Input: dimensioned drawing with shaded views. Units: mm. Origin: part minimum x, y, z. Round coordinates to 2 decimals unless told otherwise and drop trailing zeros. Loops run counter-clockwise (first coordinate to the right, second up) from the corner with the lowest first, then second, coordinate; pieces in that order, holes last. Notation, with made-up numbers: (81.25, -26.5) - (123.25, -26.5) arc R22 ccw to (123.25, 8.5) - close; hole circle Ø1 at (69.25, -26). An arc over 180 degrees is marked (long way). Answer as CSV lines item,"result".
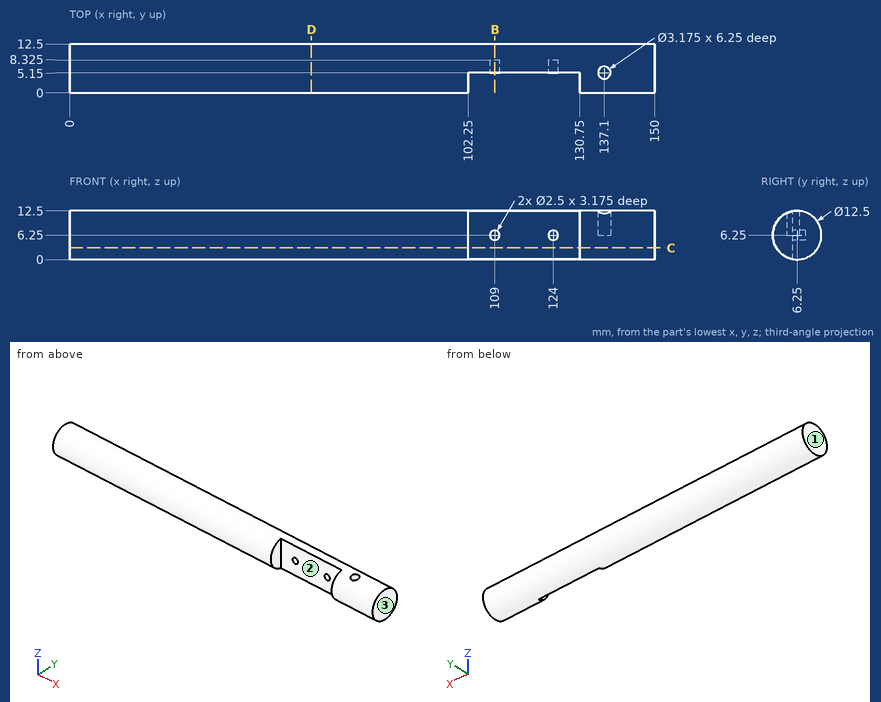
(1) Draft query along X for the marked faces 1, 2 and 3. Return one class per face: pulls with the +X half, pulls with the -X half, needs draft (parallel to the pull), parting line crosses it, or undercut.
Findings below:
face 1,"pulls with the -X half"
face 2,"undercut"
face 3,"pulls with the +X half"
(2) Material intervals for line 1 along Z through (x, y) = (109, 6.55); line 2 along X through (y, z) = (1.5, 6); line 3 along X through (y, z) = (5.25, 7.25), sorted ascending.
Findings below:
line 1,"0.01 to 5, 7.5 to 12.49"
line 2,"0 to 102.25, 130.75 to 150"
line 3,"0 to 108.25, 109.75 to 123.25, 124.75 to 135.52, 138.68 to 150"
(3) Section B-B (x = 109). Output: boundary loops of the cut face in (y, z) (3 decimals).
Findings below:
outline,"(5.15, 0.098) arc R6.25 ccw (long way) to (5.15, 12.402) - (5.15, 7.5) - (8.325, 7.5) - (8.325, 5) - (5.15, 5) - close"
(4) Section C-C (z = 3). Output: boundary loops of the cut face in (x, y), and give its area (3 significant figures).
Findings below:
outline,"(0, 0.91) - (102.25, 0.91) - (102.25, 5.15) - (130.75, 5.15) - (130.75, 0.91) - (150, 0.91) - (150, 11.59) - (0, 11.59) - close"
area,"1,480 mm2"
(5) Pin query (flat end, axial travel): P1, Ø1, axis at x = 114.5, y = 7.5, coming from the -Z side; P2, Ø2.5, axis at x = 137.1, y = 5.15, coming from the +Z side; P3, Ø4, axis at x = 57, y = 11, coming from the +Z side. Return the tip coordinate at first contact, or that it passes through.
Findings below:
P1,"z = 0.05"
P2,"z = 6.25"
P3,"z = 11.86"
(6) Section D-D (x = 62). Output: boundary loops of the cut face in (y, z), and give its area (3 significant figures).
Findings below:
outline,"circle Ø12.5 at (6.25, 6.25)"
area,"123 mm2"
